```python
from build123d import *

# Parameters (mm, degrees)
SKETCH1_R               = 50
BOSS_EXTRUDE1_DEPTH     = 40
SHELL1_T                = -5
SKETCH2_R               = 2
CUT_EXTRUDE1_DEPTH      = 79.89866919
CUT_EXTRUDE1_DEPTH_BACK = 79.89866919
SKETCH3_R               = 5
SKETCH3_R_2             = 2
BOSS_EXTRUDE2_DEPTH     = 5


with BuildPart() as part:
    # Sketch1 → Boss-Extrude1 (new body)
    with BuildSketch(Plane.XY):
        Circle(SKETCH1_R)
    extrude(amount=BOSS_EXTRUDE1_DEPTH)

    # Shell1
    shell1_openings = [part.faces().sort_by_distance(p)[0] for p in [
        (0, 0, 40),
    ]]
    offset(amount=SHELL1_T, openings=shell1_openings, kind=Kind.INTERSECTION)

    # Sketch2 → Cut-Extrude1 (cut, two sides)
    with BuildSketch(Plane.XY.offset(5)) as cut_extrude1_sk:
        Circle(SKETCH2_R)
    extrude(amount=CUT_EXTRUDE1_DEPTH, mode=Mode.SUBTRACT)
    extrude(cut_extrude1_sk.sketch, amount=-CUT_EXTRUDE1_DEPTH_BACK, mode=Mode.SUBTRACT)

    # Sketch3 → Boss-Extrude2 (add)
    with BuildSketch(Plane.XY.offset(5)):
        Circle(SKETCH3_R)
        Circle(SKETCH3_R_2, mode=Mode.SUBTRACT)
    extrude(amount=BOSS_EXTRUDE2_DEPTH)


solid = part.part
```
Can you work these out from the model? Positions are in its coordinate system, mm. A direction names the side the tool comes from. Round coordinates to 2 decimals unless told otherwise and drop trailing zeros. Order: outer loops, then holes, each group sorted by start corner. A loop starts at its lowest first (then second) coordinate and runs counter-clockwise, first axis right, second up.
(1) On a 3-axis mill with a long thin cutter (end or side, diameter ignored), from which of +Z, -Z, +X, -X, +Y, -Y can I reach the whole of each face in a straight line? I mean faces 1 (the face through (-0.1, -2.2, 10)), 2 (the face through (-41, 19, 40)). Say none if no direction works.
Results are:
face 1: +Z
face 2: +Z, +X, -X, +Y, -Y
(2) I'm going to push flat-ended pins straight in: pin 1 (1.5 mm diameter, centred on x = -2.5, z = 11.5, fed in from -Y); pin 2 (5 mm diameter, centred on x = 30, z = 30.5, fed in from -Y); pin 3 (8 mm diameter, centred on x = -8, z = 5.5, fed in from -Y). Where does each tip first touch, or does it pass through?
Results are:
pin 1: stops at y = -49.97
pin 2: stops at y = -41.76
pin 3: stops at y = -49.84
(3) We'd pull the mould along Y, two halves only. Please class faces 3 (the face through (47.69, 15.02, 19.72)), 4 (the face through (-1, -10, 0)), 5 (the face through (20.765, -39.923, 22.255)): +Y half, -Y half, draft (parallel to the pull), parting line (faces both ways), or undercut.
Results are:
face 3: parting line
face 4: draft
face 5: undercut
(4) If we section it at A-A (y = 0): Please give me the cut outline in (x, z).
Results are:
outline: (-50, 0) - (-2, 0) - (-2, 10) - (-5, 10) - (-5, 5) - (-45, 5) - (-45, 40) - (-50, 40) - close; (2, 0) - (50, 0) - (50, 40) - (45, 40) - (45, 5) - (5, 5) - (5, 10) - (2, 10) - close
(5) If I drill on L1, parallel to Y at x = 0, z = 8; L2, parallel to Y at x = 0, z = 15.5; L3, parallel to Z at x = 16.5, y = -32, over which ranges is the centre line in solid material (lowest first)?
Results are:
L1: y = -50 to -45, -5 to -2, 2 to 5, 45 to 50
L2: y = -50 to -45, 45 to 50
L3: z = 0 to 5
(6) If we section it at D-D (y = 40): Please give me the cut outline in (x, z).
Results are:
outline: (-30, 0) - (30, 0) - (30, 40) - (20.62, 40) - (20.62, 5) - (-20.62, 5) - (-20.62, 40) - (-30, 40) - close
(7) If we section it at C-C (x = 11.5): Please give me the cut outline in (y, z).
Results are:
outline: (-48.66, 0) - (48.66, 0) - (48.66, 40) - (43.51, 40) - (43.51, 5) - (-43.51, 5) - (-43.51, 40) - (-48.66, 40) - close
